Design review of the part built by this model. Coordinates are the model's own, in mm. A direction names the side the tool comes from. Coordinates: 2 decimals unless noted, no trailing zeros. Write each loop counter-clockwise with the first axis right and the second up, starting at its lowest first coordinate (ties: lowest second). Pieces come first, ordered by that corner, then holes. Notation, with made-up numbers: M -15,84.25 L 28,84.25 A14 ccw 28,106.25 Z; hole C 27.25,28.25 d4. An arc over 180 degrees is marked long. Write each question's results on one line, items separated by ' | '. Start each with the question number.
```python
from build123d import *

# Parameters (mm, degrees)
CROQUIS1_W                 = 60
CROQUIS1_H                 = 40
SALIENTE_EXTRUIR1_DEPTH    = 5
CROQUIS3_R                 = 1.5
CORTAR_EXTRUIR1_DEPTH      = 37.400549446
REDONDEO1_R                = 10
CROQUIS5_R                 = 3
CORTAR_EXTRUIR2_DEPTH      = 3.5
CROQUIS9_W                 = 10
CROQUIS9_H                 = 40
SALIENTE_EXTRUIR3_DEPTH    = 7
CORTAR_EXTRUIR5_DEPTH      = 37.728735481
CORTAR_EXTRUIR5_DEPTH_BACK = 37.728735481
CROQUIS10_R                = 1.5
CROQUIS11_R                = 3
CORTAR_EXTRUIR6_DEPTH      = 6.63
SALIENTE_EXTRUIR4_DEPTH    = 7
CORTAR_EXTRUIR7_START      = -7
CROQUIS13_R                = 8
CORTAR_EXTRUIR7_DEPTH      = 7
CORTAR_EXTRUIR8_START      = -2.25
CORTAR_EXTRUIR8_DEPTH      = 2.25


with BuildPart() as part:
    # Croquis1 → Saliente-Extruir1 (new body)
    with BuildSketch(Plane(origin=(0, 0, 0), x_dir=(0, 0, -1), z_dir=(1, 0, 0))):
        Rectangle(CROQUIS1_W, CROQUIS1_H)
    extrude(amount=SALIENTE_EXTRUIR1_DEPTH)

    # Croquis3 → Cortar-Extruir1 (cut, through all)
    with BuildSketch(Plane(origin=(5, 0, 0), x_dir=(0, 0, -1), z_dir=(1, 0, 0))):
        with Locations((-25, 15)):
            Circle(CROQUIS3_R)
        with Locations(Location((25, 15, 0), (0, 0, 180))):
            Circle(CROQUIS3_R)
        with Locations((25, -15)):
            Circle(CROQUIS3_R)
        with Locations(Location((-25, -15, 0), (0, 0, 180))):
            Circle(CROQUIS3_R)
    extrude(amount=-CORTAR_EXTRUIR1_DEPTH, mode=Mode.SUBTRACT)

    # Redondeo1
    # the kernel refuses this fillet: 10 mm, written as the material it takes off along each edge
    with BuildSketch(Plane(origin=(5, -20, 51.650635095), x_dir=(-1, 0, 0), z_dir=(0, 0, -1))) as redondeo1_piece_1:
        with BuildLine():
            CenterArc((10, 8.660254038), REDONDEO1_R, 180, 60)
            Line((0, 8.660254038), (-0.2, 8.660254038))
            Line((-0.2, 8.660254038), (-0.2, 0))
            Line((-0.2, 0), (0, -0.2))
            ThreePointArc((0, -0.2), (2.5, -0.2), (4.9, -0.173205081))
            Line((4.9, -0.173205081), (5, 0))
        make_face()
    extrude(amount=103.301270189, mode=Mode.SUBTRACT)
    with BuildSketch(Plane(origin=(5, 20, -51.650635095), x_dir=(0, -1, 0), z_dir=(0, 0, 1))) as redondeo1_piece_2:
        with BuildLine():
            CenterArc((8.660254038, -10), REDONDEO1_R, 90, 60)
            Line((0, -5), (-0.173205081, -4.9))
            ThreePointArc((-0.173205081, -4.9), (-0.2, -2.5), (-0.2, 0))
            Line((-0.2, 0), (0, 0.2))
            Line((0, 0.2), (8.660254038, 0.2))
            Line((8.660254038, 0.2), (8.660254038, 0))
        make_face()
    extrude(amount=103.301270189, mode=Mode.SUBTRACT)
    with BuildSketch(Plane(origin=(5, 41.650635095, 30), x_dir=(-1, 0, 0), z_dir=(0, -1, 0)), Plane(origin=(5, -41.650635095, -30), x_dir=(-1, 0, 0), z_dir=(0, 1, 0))) as redondeo1_piece_3:
        with BuildLine():
            CenterArc((10, 8.660254038), REDONDEO1_R, 180, 60)
            Line((0, 8.660254038), (-0.2, 8.660254038))
            Line((-0.2, 8.660254038), (-0.2, 0))
            Line((-0.2, 0), (0, -0.2))
            ThreePointArc((0, -0.2), (2.5, -0.2), (4.9, -0.173205081))
            Line((4.9, -0.173205081), (5, 0))
        make_face()
    extrude(amount=83.301270189, mode=Mode.SUBTRACT)

    # Croquis5 → Cortar-Extruir2 (cut)
    with BuildSketch(Plane(origin=(5, 0, 0), x_dir=(0, 0, -1), z_dir=(1, 0, 0))):
        with Locations((-25, 15)):
            Circle(CROQUIS5_R)
        with Locations((25, 15)):
            Circle(CROQUIS5_R)
        with Locations((25, -15)):
            Circle(CROQUIS5_R)
        with Locations((-25, -15)):
            Circle(CROQUIS5_R)
    extrude(amount=-CORTAR_EXTRUIR2_DEPTH, mode=Mode.SUBTRACT)

    # Croquis9 → Saliente-Extruir3 (add)
    with BuildSketch(Plane.ZY):
        with Locations((-25, 0)):
            Rectangle(CROQUIS9_W, CROQUIS9_H)
        with Locations((25, 0)):
            Rectangle(CROQUIS9_W, CROQUIS9_H)
    extrude(amount=SALIENTE_EXTRUIR3_DEPTH)

    # Croquis10 → Cortar-Extruir5 (cut, two sides: drawn at the far end of the back side and taken through both)
    with BuildSketch(Plane(origin=(0, 0, 0), x_dir=(0, 0, -1), z_dir=(1, 0, 0)).offset(-CORTAR_EXTRUIR5_DEPTH_BACK)):
        with Locations((-25, -15)):
            Circle(CROQUIS10_R)
        with Locations((25, -15)):
            Circle(CROQUIS10_R)
        with Locations((25, 15)):
            Circle(CROQUIS10_R)
        with Locations((-25, 15)):
            Circle(CROQUIS10_R)
    extrude(amount=CORTAR_EXTRUIR5_DEPTH + CORTAR_EXTRUIR5_DEPTH_BACK, mode=Mode.SUBTRACT)

    # Croquis11 → Cortar-Extruir6 (cut)
    with BuildSketch(Plane(origin=(1.5, 0, 0), x_dir=(0, 0, -1), z_dir=(1, 0, 0))):
        with Locations((-25, 15)):
            Circle(CROQUIS11_R)
        with Locations((25, -15)):
            Circle(CROQUIS11_R)
        with Locations((-25, -15)):
            Circle(CROQUIS11_R)
        with Locations((25, 15)):
            Circle(CROQUIS11_R)
    extrude(amount=-CORTAR_EXTRUIR6_DEPTH, mode=Mode.SUBTRACT)

    # Croquis12 → Saliente-Extruir4 (add)
    with BuildSketch(Plane.ZY):
        with BuildLine():
            Line((-5, 6.244997998), (-5, 10.255002002))
            ThreePointArc((-5, 10.255002002), (-7.804685433, 14.743046588), (-7.193747285, 20))
            Line((-7.193747285, 20), (7.193747285, 20))
            ThreePointArc((7.193747285, 20), (7.804685433, 14.743046588), (5, 10.255002002))
            Line((5, 10.255002002), (5, 6.244997998))
            ThreePointArc((5, 6.244997998), (0, -8), (-5, 6.244997998))
        make_face()
    extrude(amount=SALIENTE_EXTRUIR4_DEPTH)

    # Croquis13 → Cortar-Extruir7 (cut)
    with BuildSketch(Plane.ZY.offset(7).offset(CORTAR_EXTRUIR7_START)):
        Circle(CROQUIS13_R)
    extrude(amount=CORTAR_EXTRUIR7_DEPTH, mode=Mode.SUBTRACT)

    # Croquis15 → Cortar-Extruir8 (cut)
    with BuildSketch(Plane.ZY.offset(7).offset(CORTAR_EXTRUIR8_START)):
        with BuildLine():
            Line((5, 6.244997998), (5, 10.255002002))
            ThreePointArc((5, 10.255002002), (7.804685433, 14.743046588), (7.193747285, 20))
            Line((7.193747285, 20), (-7.193747285, 20))
            ThreePointArc((-7.193747285, 20), (-7.804685433, 14.743046588), (-5, 10.255002002))
            Line((-5, 10.255002002), (-5, 6.244997998))
            ThreePointArc((-5, 6.244997998), (0, 8), (5, 6.244997998))
        make_face()
    extrude(amount=CORTAR_EXTRUIR8_DEPTH, mode=Mode.SUBTRACT)


solid = part.part
```
Item 1: We need section D-D on x = 0.75. State the section outline as (y, z) points.
Item 2: We need section A-A on x = -3.25. State the section outline as (y, z) points (3 decimals).
Item 3: We need section B-B on z = 25. State the section outline as (x, y) points, then the cut area to 3 significant figures.
Item 4: We need section C-C on y = 15. State the section outline as (x, z) points.
Item 5: Wall thickness on L1, parallel to Z at x = -6.3, y = 15; L2, parallel to Y at x = -1.5, z = 25; L3, parallel to Z at x = -0.5, y = -6.5: over which ranges is each line inside the solid? List them lowest first.
Item 6: Insertion check: pin 1 Ø1.8 at (y, z) = (16.5, -25) entering from +X; pin 2 Ø1.5 at (x, y) = (2.5, 3) entering from -Z; pin 3 Ø2.5 at (y, z) = (-15, 25) entering from +X; pin 4 Ø4 at (y, z) = (10.5, 2) entering from -X. Each pin has a flat end and moves straight along its axis. Give the tip position at first contact, or say it passes through.
Item 7: For faces 1 (the flat face through (-2, 8, -5)), 2 (the flat face through (-7, 0, 25)), 3 (the flat face through (-3, 0, -20)), 4 (the flat face through (-5.13, 13.7, 23.7)), 5 (the cylindrical face through (-2.342, 14.669, -7.788)), list the 3-axis set-ups (+Z, -Z, +X, -X, +Y, -Y) from which the entire face can be reached by the end or side of a thin tool; tool diameter is ignored.
Item 8: Draft analysis for pull direction Z (two halves, no side actions). For faces 6 (the flat face through (-7, 0, -25)), 7 (the cylindrical face through (-6.08, -14.93, 26.5)), state which applies: released by +Z, released by -Z, zero draft, split by the parting line, or undercut.
Answer:
1) outline: M -19.52,-29.52 L 19.52,-29.52 L 19.52,29.52 L -19.52,29.52 Z; hole C -15,-25 d6; hole C -15,25 d6; hole C 15,-25 d6; hole C 15,25 d6
2) outline: M -20,-30 L 20,-30 L 20,-20 L -20,-20 Z; M -20,20 L 20,20 L 20,30 L -20,30 Z; M 6.245,-5 L 10.255,-5 A8 ccw 20,-7.194 L 20,7.194 A8 ccw 10.255,5 L 6.245,5 A8 cw Z; hole C -15,-25 d6; hole C -15,25 d6; hole C 15,-25 d6; hole C 15,25 d6
3) outline: M -7,-20 L 0,-20 A10 ccw 2.46,-18 L -5.13,-18 L -5.13,-16.5 L -7,-16.5 Z; M -7,-13.5 L -5.13,-13.5 L -5.13,-12 L 4.31,-12 L 4.31,12 L -5.13,12 L -5.13,13.5 L -7,13.5 Z; M -7,16.5 L -5.13,16.5 L -5.13,18 L 2.46,18 A10 ccw 0,20 L -7,20 Z | area: 316 mm^2
4) outline: M -7,-30 L 0,-30 A10 ccw 2.46,-28 L -5.13,-28 L -5.13,-26.5 L -7,-26.5 Z; M -7,-23.5 L -5.13,-23.5 L -5.13,-22 L 4.31,-22 L 4.31,22 L -5.13,22 L -5.13,23.5 L -7,23.5 L -7,20 L 0,20 L 0,7.86 L -4.75,7.86 L -4.75,-7.86 L 0,-7.86 L 0,-20 L -7,-20 Z; M -7,26.5 L -5.13,26.5 L -5.13,28 L 2.46,28 A10 ccw 0,30 L -7,30 Z
5) L1: z = -30 to -26.5, -23.5 to -20, 20 to 23.5, 26.5 to 30 | L2: y = -20 to -18, -12 to 12, 18 to 20 | L3: z = -30 to -20, 20 to 30
6) pin 1: stops at x = -5.13 | pin 2: stops at z = -28.72 | pin 3: passes through | pin 4: stops at x = -4.75
7) face 1: -X, -Y | face 2: +Z, -Z, -X, +Y, -Y | face 3: -X, +Y, -Y | face 4: +X | face 5: -X
8) face 6: zero draft | face 7: undercut
